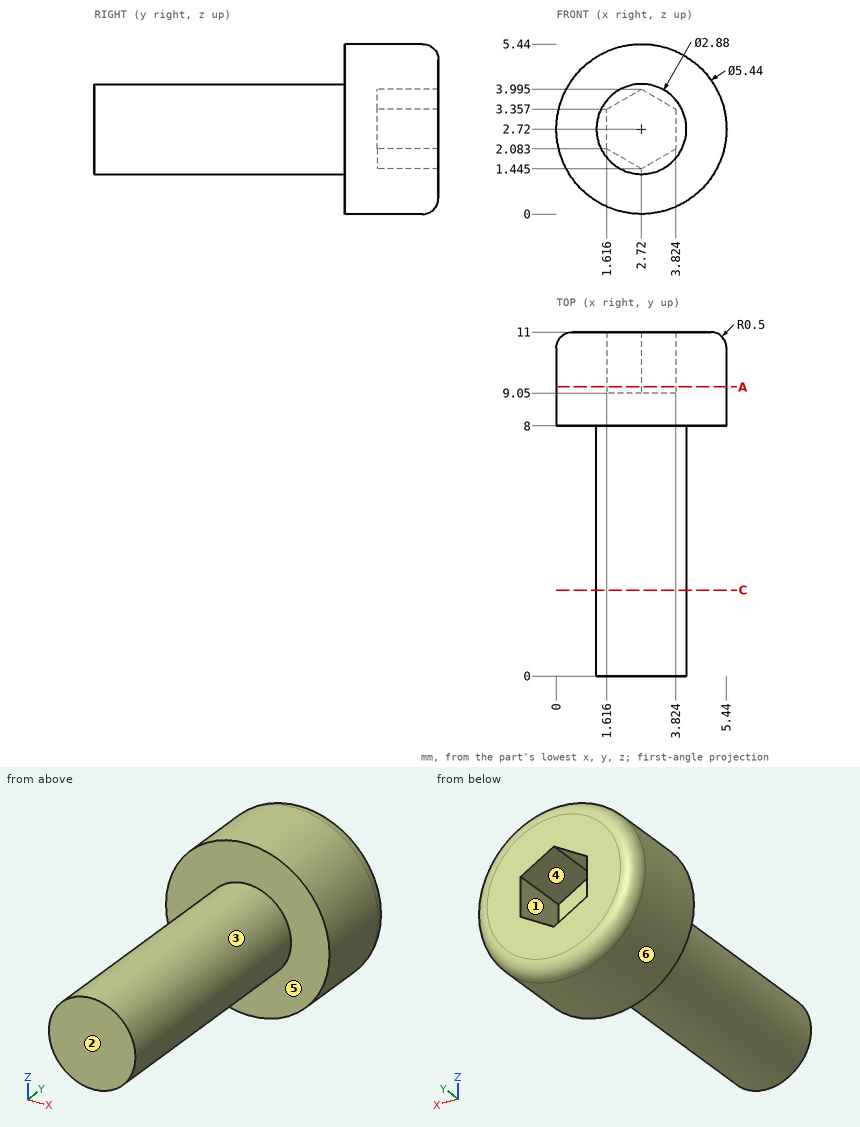
The figure shows three views and two pictorial views of one solid part (mm, origin at its lowest corner). Answer the questions. A direction names the side the tool comes from. Coordinates: 2 decimals unless noted, no trailing zeros. Write each loop counter-clockwise with the first axis right and the second up, starting at its lowest first coordinate (ties: lowest second). Pieces come first, ordered by that corner, then holes. Notation, with made-up numbers: (-17.75, 4) -> (0.25, 4) arc R24 ccw to (0.25, 32) -> close; hole circle Ø5 at (33, -23.75). An arc over 180 degrees is marked (long way). Answer as a JSON object with one key per item and string values.
Q1. Flat-ended cylindrical pins translate along their axes: pin 1 Ø3 at (x, y) = (4, 5.5) entering from -Z; pin 2 Ø1 at (x, y) = (2.5, 2) entering from +Z; pin 3 Ø1.6 at (x, z) = (2.5, 2.5) entering from -Y; pin 4 Ø0.7 at (x, z) = (3, 2.5) entering from +Y. Find the tip coordinate at first contact, or state that the pin passes through.
The answers:
{"pin 1": "stops at z = 1.28", "pin 2": "stops at z = 4.16", "pin 3": "stops at y = 0", "pin 4": "stops at y = 9.05"}
Q2. The part is cut by section C-C on y = 2.75. Give the vertices of the cut face in (x, z).
The answers:
{"outline": "circle Ø2.88 at (2.72, 2.72)"}
Q3. Determine the mould class of the marked faces 1, 2 and 3 for opening direction Z: pulls with the +Z half, pulls with the -Z half, needs draft (parallel to the pull), parting line crosses it, or undercut.
The answers:
{"face 1": "undercut", "face 2": "needs draft", "face 3": "parting line crosses it"}
Q4. A tool of negligible diameter and unlimited length cuts with its end or side. For the marked faces 4, 5 and 6, from which of +Z, -Z, +X, -X, +Y, -Y can it reach the whole face along a straight path? Write none if from no direction.
The answers:
{"face 4": "+Y", "face 5": "-Y", "face 6": "+Y, -Y"}
Q5. The part is cut by section A-A on y = 9.25. Give the vertices of the cut face in (x, z) (1 decimal), then the cut area to 3 significant figures.
The answers:
{"outline": "circle Ø5.4 at (2.7, 2.7); hole (1.6, 2.1) -> (2.7, 1.4) -> (3.8, 2.1) -> (3.8, 3.4) -> (2.7, 4) -> (1.6, 3.4) -> close", "area": "19.0 mm2"}
Q6. Consider line 1 (Y direction, x = 3.4, z = 4.75); line 2 (Y direction, x = 3.55, z = 2.7); line 3 (X direction, y = 9.5, z = 3.9) (1 decimal). Determine where each line is inside the solid, lowest interval first. Write a range as [from, to].
The answers:
{"line 1": "y = [8, 11]", "line 2": "y = [0, 9.05]", "line 3": "x = [0.3, 2.6], [2.9, 5.2]"}
